from build123d import *

# Parameters (mm, degrees)
CROQUIS1_R              = 6.7
CROQUIS1_R_2            = 5.9
SALIENTE_EXTRUIR1_DEPTH = 4.2
CROQUIS3_R              = 7.4
CROQUIS3_R_2            = 5.9
SALIENTE_EXTRUIR2_DEPTH = 2
REDONDEO1_R             = 0.5
CHAFL_N1_SIZE           = 0.7
CROQUIS2_W              = 20.515822
CROQUIS2_H              = 3.3
CORTAR_EXTRUIR1_DEPTH   = 3.9


with BuildPart() as part:
    # Croquis1 → Saliente-Extruir1 (new body)
    with BuildSketch(Plane.XY):
        Circle(CROQUIS1_R)
        Circle(CROQUIS1_R_2, mode=Mode.SUBTRACT)
    extrude(amount=SALIENTE_EXTRUIR1_DEPTH)

    # Croquis3 → Saliente-Extruir2 (add)
    with BuildSketch(Plane(origin=(0, 0, 0), x_dir=(-1, 0, 0), z_dir=(0, 0, -1))):
        Circle(CROQUIS3_R)
        with Locations(Location((0, 0, 0), (0, 0, 180))):
            Circle(CROQUIS3_R_2, mode=Mode.SUBTRACT)
    extrude(amount=-SALIENTE_EXTRUIR2_DEPTH)

    # Redondeo1
    redondeo1_edges = [part.edges().sort_by_distance(p)[0] for p in [
        (-6.7, 0, 4.2),
    ]]
    fillet(redondeo1_edges, radius=REDONDEO1_R)

    # Chaflán1
    chafl_n1_edges = [part.edges().sort_by_distance(p)[0] for p in [
        (-6.7, 0, 2),
    ]]
    chamfer(chafl_n1_edges, length=CHAFL_N1_SIZE - 0.0001)  # a hair under: the kernel refuses the full size

    # Croquis2 → Cortar-Extruir1 (cut)
    with BuildSketch(Plane.XY.offset(4.2)):
        Rectangle(CROQUIS2_W, CROQUIS2_H)
    extrude(amount=-CORTAR_EXTRUIR1_DEPTH, mode=Mode.SUBTRACT)


solid = part.part
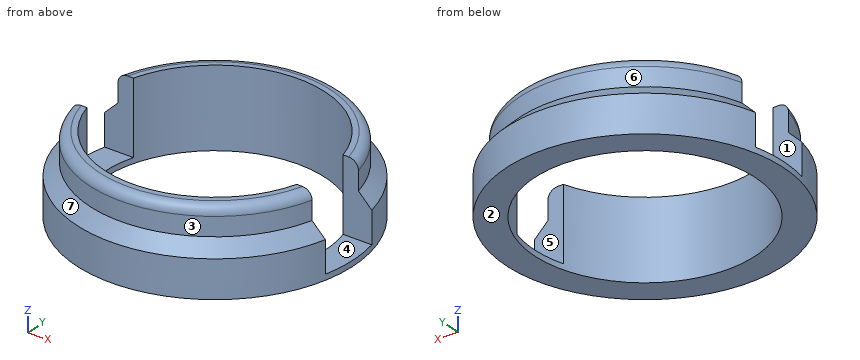
Source: CAD feature listing. Evaluate the final solid. Frame: model axes, mm. Face numbers are marked on the shaded views. A direction names the side the tool comes from. Coordinates: 2 decimals unless noted, no trailing zeros. Order: outer loops, then holes, each group sorted by start corner. A loop starts at its lowest first (then second) coordinate and runs counter-clockwise, first axis right, second up.
Item 1: Material intervals for line 1 (Y direction, x = 0, z = 3.1); line 2 (Z direction, x = -6, y = 0); line 3 (Y direction, x = 4, z = 2.35), sorted ascending.
Output values:
line 1: y = -6.7 to -5.9, 5.9 to 6.7
line 2: z = 0 to 0.3
line 3: y = -5.81 to -4.34, 4.34 to 5.81
Item 2: Set-up query: the marked faces 1, 2 and 3. Return all of +Z, -Z, +X, -X, +Y, -Y with unobstructed straight access to the full face (end or side cutting, diameter ignored); none if empty.
Output values:
face 1: +Z, +X, -X
face 2: -Z, +X, -X, +Y, -Y
face 3: +Z, -Y
Item 3: Cut plane B-B (y = 0). Return loops of the section in (x, z), plus the area to 3 significant figures.
Output values:
outline: (-7.4, 0) - (-5.9, 0) - (-5.9, 0.3) - (-7.4, 0.3) - close; (5.9, 0) - (7.4, 0) - (7.4, 0.3) - (5.9, 0.3) - close
area: 0.900 mm2
Item 4: Cut plane A-A (z = 3.3). Return loops of the section in (x, y), plus the area to 3 significant figures.
Output values:
outline: (-6.49, -1.65) arc R6.7 ccw to (6.49, -1.65) - (5.66, -1.65) arc R5.9 cw to (-5.66, -1.65) - close; (-6.49, 1.65) - (-5.66, 1.65) arc R5.9 cw to (5.66, 1.65) - (6.49, 1.65) arc R6.7 ccw to start
area: 26.3 mm2
Item 5: First-contact query: P1, Ø1.5, axis at y = 4, z = 3, coming from the -X side; P2, Ø1.4, axis at x = 7, y = -0.5, coming from the +Z side; P3, Ø1.2, axis at x = 6.5, z = 1.5, coming from the +Y side. Flat tips, straight axial feed; report the tip coordinate or a pass-through.
Output values:
P1: stops at x = -6.05
P2: stops at z = 0.3
P3: stops at y = 4.47
Item 6: Pull-direction query (Y, two-part tool) for the marked faces 4, 5, 6 and 7; classes: pulls with the +Y half, pulls with the -Y half, needs draft (parallel to the pull), parting line crosses it, or undercut.
Output values:
face 4: undercut
face 5: undercut
face 6: pulls with the +Y half
face 7: pulls with the -Y half
